Source: CAD feature listing. Evaluate the final solid. Frame: model axes, mm. A direction names the side the tool comes from. Give positions to 0.01 mm unless a question says otherwise; leave off trailing zeros. Loops run counter-clockwise (first coordinate to the right, second up) from the corner with the lowest first, then second, coordinate; pieces in that order, holes last. Notation, with made-up numbers: M 7.5,49 L 43.5,49 A16 cw 43.5,67 Z; hole C 80.25,23.25 d2. An arc over 180 degrees is marked long. Write item = value, one per line.
from build123d import *

# Parameters (mm, degrees)
F0_W     = 12.7
F0_H     = 7.9375
F2_R     = 3.175
F3_DEPTH = 6.35


with BuildPart() as f1:
    # F0 (on Right) → F1 (revolve)
    with BuildSketch(Plane.YZ):
        with Locations((9.525, 8.73125)):
            Rectangle(F0_W, F0_H)
        Polygon((0, 4.7625), (3.175, 4.7625), (3.175, 12.7), (3.175, 15.875), (0, 15.875), align=None)
        Polygon((15.875, 4.7625), (19.05, 4.7625), (19.05, 15.875), (15.875, 15.875), (15.875, 12.7), align=None)
    revolve(axis=Axis((0, 9.525, 0), (0, 1, 0)))

    # F2 (on Front) → F3 (join)
    with BuildSketch(Plane.XZ):
        with Locations((9.525, 0)):
            Circle(F2_R)
    extrude(amount=F3_DEPTH)


solid = f1.part
1. Pull-direction query (Y, two-part tool) for faces 4 (the flat face through (11, 3.175, 7)), 5 (the flat face through (4, 19.05, -3)), 6 (the cylindrical face through (-15.497, 17.44, -3.441)), 7 (the flat face through (9, -6.35, 0)); classes: +Y half, -Y half, draft (parallel to the pull), parting line (faces both ways), or undercut.
Derived:
face_4 = undercut
face_5 = +Y half
face_6 = draft
face_7 = -Y half
2. Material intervals for probe 1 along X at (y, z) = (5.25, 0); probe 2 along Y at (x, z) = (-11, -8.5) (3 decimals); probe 3 along Y at (x, z) = (-2, 10), sorted ascending. Write a range as from..to.
Derived:
probe_1 = -12.7..-4.76, 4.76..12.7
probe_2 = 0..3.175, 15.875..19.05
probe_3 = 0..19.05
3. Reachability of faces 1 (the flat face through (11, 15.875, -7)), 2 (the cylindrical face through (-2.9, 9.66, -3.78)), 3 (the cylindrical face through (12.458, -3.131, -1.216)) from +Z, -Z, +X, -X, +Y, -Y: full face, straight path, thin tool, end or side. Return the list, or none.
Derived:
face_1 = none
face_2 = +Y, -Y
face_3 = -Y
4. Cut plane C-C, the plane y = 10. Return the cut outline in (x, z) (1 decimal).
Derived:
outline = C 0,0 d25.4; hole C 0,0 d9.5
5. First-contact query: pin 1 Ø12 at (x, y) = (7.5, 14.5) entering from -Z; pin 2 Ø10 at (x, z) = (0, 7.5) entering from -Y; pin 3 Ø8 at (x, y) = (10.5, 1) entering from +Z. Flat tips, straight axial feed; report the tip coordinate or a pass-through.
Derived:
pin_1 = -15.79
pin_2 = 0
pin_3 = 14.48
6. Cut plane D-D, the plane x = 9. Return the cut outline in (y, z) (3 decimals).
Derived:
outline = M -6.35,-3.131 L 0,-3.131 L 0,-13.077 L 3.175,-13.077 L 3.175,-8.96 L 15.875,-8.96 L 15.875,-13.077 L 19.05,-13.077 L 19.05,13.077 L 15.875,13.077 L 15.875,8.96 L 3.175,8.96 L 3.175,13.077 L 0,13.077 L 0,3.131 L -6.35,3.131 Z
